from build123d import *

# Parameters (mm, degrees)
CHAMBRAGE_POUR_VIS_T_TE_CYLINDRIQUE_D           = 4.5
CHAMBRAGE_POUR_VIS_T_TE_CYLINDRIQUE_CBORE_D     = 8
CHAMBRAGE_POUR_VIS_T_TE_CYLINDRIQUE_CBORE_DEPTH = 4
R_P_TITION_CIRCULAIRE1_COUNT                    = 3


with BuildPart() as part:
    # Esquisse1 → Révolution1 (revolve)
    with BuildSketch(Plane.XY, mode=Mode.PRIVATE) as r_volution1_sk:
        Polygon((20, 6), (20, 0), (33, 0), (33, 8), (23.5, 8), (23.5, 6), align=None)
    revolve(r_volution1_sk.sketch.rotate(Axis((0, 31.17754591, 0), (0, -1, 0)), 90), axis=Axis((0, 31.17754591, 0), (0, -1, 0)))

    # Chambrage pour vis à tête cylindrique à 6 pans creux (ou vis CHC) M41 (through all)
    with Locations(Plane.XZ):
        with Locations((28.5, 0)):
            chambrage_pour_vis_t_te_cylindrique = CounterBoreHole(CHAMBRAGE_POUR_VIS_T_TE_CYLINDRIQUE_D / 2, CHAMBRAGE_POUR_VIS_T_TE_CYLINDRIQUE_CBORE_D / 2, CHAMBRAGE_POUR_VIS_T_TE_CYLINDRIQUE_CBORE_DEPTH)

    # Répétition circulaire1: Chambrage pour vis à tête cylindrique à 6 pans creux (ou vis CHC) M41 ×3 about axis
    r_p_tition_circulaire1_axis = Axis((0, 0, 0), (0, 1, 0))
    for i in range(1, R_P_TITION_CIRCULAIRE1_COUNT):
        add(chambrage_pour_vis_t_te_cylindrique.rotate(r_p_tition_circulaire1_axis, i * 360 / R_P_TITION_CIRCULAIRE1_COUNT), mode=Mode.SUBTRACT)


solid = part.part
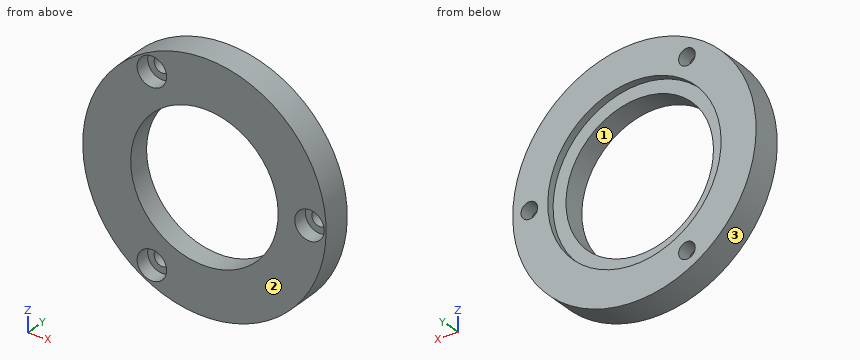
Source: CAD feature listing. Evaluate the final solid. Frame: model axes, mm. Face numbers are marked on the shaded views. Round coordinates to 2 decimals unless told otherwise and drop trailing zeros. Loops run counter-clockwise (first coordinate to the right, second up) from the corner with the lowest first, then second, coordinate; pieces in that order, holes last.
Q1. Ray query, line 1 (Z direction, x = -14.25, y = 2.6); line 2 (X direction, y = 3, z = -1.5); line 3 (Z direction, x = -14.25, y = 5.3). Return the intervals inside material, ascending.
Q2. First-contact query: P1, Ø1, axis at y = 3.5, z = -6, coming from the -X side; P2, Ø6, axis at x = 28.5, z = 0, coming from the -Y side; P3, Ø4, axis at x = 13, y = 4, coming from the +Z side. Flat tips, straight axial feed; report the tip coordinate or a pass-through.
Q3. Mould query, pull axis Z, two halves, no side actions, for the marked faces 1, 2 and 3. Classes: pulls with the +Z half, pulls with the -Z half, needs draft (parallel to the pull), parting line crosses it, or undercut.
Q4. Section B-B, the plane z = 0. Return loops of the section in (x, y), plus the area to 3 significant figures.
Q5. Section A-A, the plane x = 0. Return loops of the section in (y, z), plus the area to 3 significant figures.
Q6. Section C-C, the plane z = 10.5. Return loops of the section in (x, y).
Q7. Section D-D, the plane y = 7.25. Return loops of the section in (x, z) (3 decimals), plus the area to 3 significant figures.
Solutions:
1. line 1: z = -29.76 to -28.68, -20.68 to -14.03, 14.03 to 20.68, 28.68 to 29.76
1. line 2: x = -32.97 to -19.94, 19.94 to 24.79, 32.21 to 32.97
1. line 3: z = -29.76 to -26.93, -22.43 to -14.03, 14.03 to 22.43, 26.93 to 29.76
2. P1: stops at x = -32.54
2. P2: stops at y = 4
2. P3: stops at z = 31.11
3. face 1: undercut
3. face 2: needs draft
3. face 3: parting line crosses it
4. outline: (-33, 0) - (-20, 0) - (-20, 6) - (-23.5, 6) - (-23.5, 8) - (-33, 8) - close; (20, 0) - (24.5, 0) - (24.5, 4) - (26.25, 4) - (26.25, 8) - (23.5, 8) - (23.5, 6) - (20, 6) - close; (30.75, 4) - (32.5, 4) - (32.5, 0) - (33, 0) - (33, 8) - (30.75, 8) - close
4. area: 144 mm2
5. outline: (0, -33) - (8, -33) - (8, -23.5) - (6, -23.5) - (6, -20) - (0, -20) - close; (0, 20) - (6, 20) - (6, 23.5) - (8, 23.5) - (8, 33) - (0, 33) - close
5. area: 194 mm2
6. outline: (-31.28, 0) - (-17.02, 0) - (-17.02, 6) - (-21.02, 6) - (-21.02, 8) - (-31.28, 8) - close; (17.02, 0) - (31.28, 0) - (31.28, 8) - (21.02, 8) - (21.02, 6) - (17.02, 6) - close
7. outline: circle Ø66 at (0, 0); hole circle Ø47 at (0, 0); hole circle Ø4.5 at (-14.25, -24.682); hole circle Ø4.5 at (-14.25, 24.682); hole circle Ø4.5 at (28.5, 0)
7. area: 1,640 mm2
